Check sheet for the modelled part. Datum: model origin and axes. Units: mm. Face numbers are marked on the shaded views. A direction names the side the tool comes from. Round coordinates to 2 decimals unless told otherwise and drop trailing zeros. Loops run counter-clockwise (first coordinate to the right, second up) from the corner with the lowest first, then second, coordinate; pieces in that order, holes last. Notation, with made-up numbers: (18, -8) -> (44, -8) arc R18 ccw to (44, 22) -> close; hole circle Ø7 at (30, 34.5). An arc over 180 degrees is marked (long way). One line per question, with ' | ' between items.
```python
from build123d import *

# Parameters (mm, degrees)
SKETCH1_R           = 5.25
BOSS_EXTRUDE1_DEPTH = 42
SKETCH2_R           = 2.5
BOSS_EXTRUDE2_DEPTH = 2
FILLET1_R           = 1


with BuildPart() as part:
    # Sketch1 → Boss-Extrude1 (new body)
    with BuildSketch(Plane(origin=(0, 0, 0), x_dir=(1, 0, 0), z_dir=(0, 1, 0))):
        Circle(SKETCH1_R)
    extrude(amount=BOSS_EXTRUDE1_DEPTH)

    # Sketch2 → Boss-Extrude2 (add)
    with BuildSketch(Plane(origin=(0, 42, 0), x_dir=(1, 0, 0), z_dir=(0, 1, 0))):
        Circle(SKETCH2_R)
    extrude(amount=BOSS_EXTRUDE2_DEPTH)

    # Fillet1
    fillet1_edges = [part.edges().sort_by_distance(p)[0] for p in [
        (-5.25, 0, 0),
        (-5.25, 42, 0),
        (-2.5, 44, 0),
    ]]
    fillet(fillet1_edges, radius=FILLET1_R)


solid = part.part
```
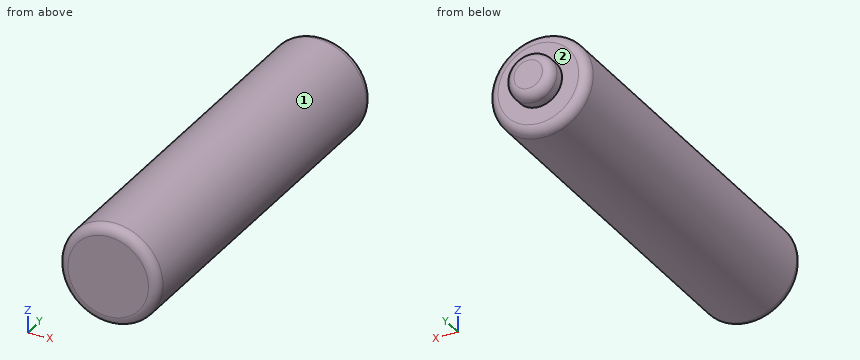
(1) Set-up check for the marked faces 1 and 2: record each of +Z, -Z, +X, -X, +Y, -Y from which the full face is reachable in a straight line by a thin tool's end or side.
Answer:
face 1: +Y, -Y | face 2: +Y
(2) Sectioned sample at B-B, the plane z = 0. Record the cut outline in (x, y).
Answer:
outline: (-5.25, 1) arc R1 ccw to (-4.25, 0) -> (4.25, 0) arc R1 ccw to (5.25, 1) -> (5.25, 41) arc R1 ccw to (4.25, 42) -> (2.5, 42) -> (2.5, 43) arc R1 ccw to (1.5, 44) -> (-1.5, 44) arc R1 ccw to (-2.5, 43) -> (-2.5, 42) -> (-4.25, 42) arc R1 ccw to (-5.25, 41) -> close
(3) Go/stop test with flat-tipped pins: pin 1 (1 mm diameter, centred on y = 8.5, z = -1.5, fed in from +X); pin 2 (4 mm diameter, centred on y = 22, z = -4, fed in from +X); pin 3 (2 mm diameter, centred on y = 37.5, z = 4, fed in from +X). Record where each tip stops, or that it passes through.
Answer:
pin 1: stops at x = 5.15 | pin 2: stops at x = 4.85 | pin 3: stops at x = 4.31
(4) Sectioned sample at C-C, the plane y = 39. Record the cut outline in (x, z).
Answer:
outline: circle Ø10.5 at (0, 0)
(5) Scan lines: probe 1 along Y at (x, z) = (-2.75, 0.25); probe 2 along X at (y, z) = (32, 0.25); probe 3 along Y at (x, z) = (-1.5, 0.5). Record each from-to range of solid material in increasing order.
Answer:
probe 1: y = 0 to 42 | probe 2: x = -5.24 to 5.24 | probe 3: y = 0 to 44
(6) Sectioned sample at A-A, the plane x = 0. Record the cut outline in (y, z), and give its area (3 significant figures).
Answer:
outline: (0, -4.25) arc R1 ccw to (1, -5.25) -> (41, -5.25) arc R1 ccw to (42, -4.25) -> (42, -2.5) -> (43, -2.5) arc R1 ccw to (44, -1.5) -> (44, 1.5) arc R1 ccw to (43, 2.5) -> (42, 2.5) -> (42, 4.25) arc R1 ccw to (41, 5.25) -> (1, 5.25) arc R1 ccw to (0, 4.25) -> close | area: 450 mm2
